The figure shows three views and two pictorial views of one solid part (mm, origin at its lowest corner). Answer the questions. A direction names the side the tool comes from. Give positions to 0.01 mm unless a question says otherwise; leave off trailing zeros. Write each loop counter-clockwise with the first axis right and the second up, starting at its lowest first coordinate (ties: lowest second). Pieces come first, ordered by that corner, then holes. Notation, with made-up numbers: (81.5, -9) - (139.5, -9) arc R23 ccw to (139.5, 15) - close; hole circle Ø2 at (85, 33). An arc over 180 degrees is marked (long way). Use CSV: the item, a comma, the result in double quotes. Start each with the question number.
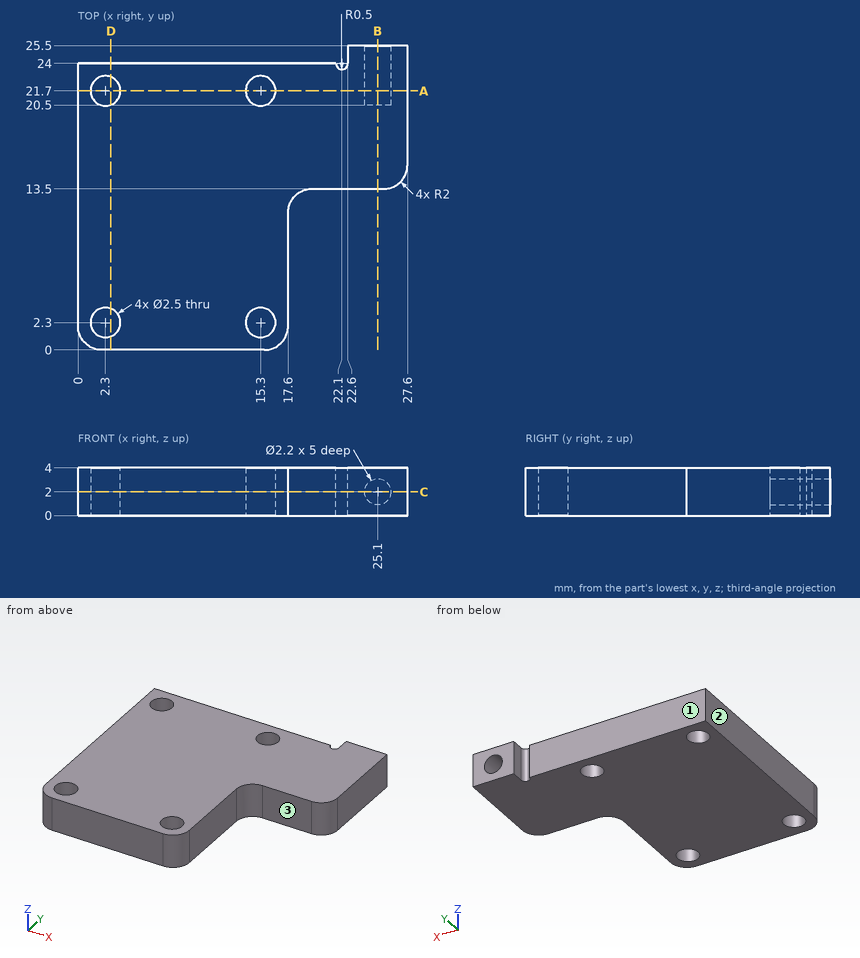
(1) The part is cut by section A-A on y = 21.7. Write down the section's boundary in (x, z), plus the area to 3 significant figures.
(2) The part is cut by section C-C on z = 2. Write down the section's boundary in (x, y), plus the area to 3 significant figures.
(3) The part is cut by section D-D on x = 2.75. Write down the section's boundary in (y, z), plus the area to 3 significant figures.
(4) The part is cut by section B-B on x = 25.1. Write down the section's boundary in (y, z), plus the area to 3 significant figures.
(5) Consider probe 1 along Y at (x, z) = (2.3, 2.7); probe 2 along X at (y, z) = (24.25, 2); probe 3 along X at (y, z) = (9.25, 0.65). Determine where each line is inside the solid, lowest interval first.
(6) Given P1, Ø1.5, axis at x = 19, z = 0.5, coming from the -Y side; P2, Ø2, axis at x = 15.3, y = 2.3, coming from the +Z side; P3, Ø1.8, axis at x = 25.1, z = 2, coming from the +Y side, each flat-ended and moving along its own axis, determine where each tip first touches the part or whether it passes through.
(7) Which of the six approach directions +Z, -Z, +X, -X, +Y, -Y give full straight-line access (tool end or side, diameter ignored) to the marked faces 1, 2 and 3?
Reported:
1,outline,"(0, 0) - (1.05, 0) - (1.05, 4) - (0, 4) - close; (3.55, 0) - (14.05, 0) - (14.05, 4) - (3.55, 4) - close; (16.55, 0) - (27.6, 0) - (27.6, 4) - (16.55, 4) - close; hole circle Ø2.2 at (25.1, 2)"
1,area,"86.6 mm²"
2,outline,"(0, 2) arc R2 ccw to (2, 0) - (15.6, 0) arc R2 ccw to (17.6, 2) - (17.6, 11.5) arc R2 cw to (19.6, 13.5) - (25.6, 13.5) arc R2 ccw to (27.6, 15.5) - (27.6, 25.5) - (26.2, 25.5) - (26.2, 20.5) - (24, 20.5) - (24, 25.5) - (22.6, 25.5) - (22.6, 24) arc R0.5 cw to (21.6, 24) - (0, 24) - close; hole circle Ø2.5 at (2.3, 2.3); hole circle Ø2.5 at (2.3, 21.7); hole circle Ø2.5 at (15.3, 2.3); hole circle Ø2.5 at (15.3, 21.7)"
2,area,"502 mm²"
3,outline,"(0, 0) - (1.13, 0) - (1.13, 4) - (0, 4) - close; (3.47, 0) - (20.53, 0) - (20.53, 4) - (3.47, 4) - close; (22.87, 0) - (24, 0) - (24, 4) - (22.87, 4) - close"
3,area,"77.3 mm²"
4,outline,"(13.5, 0) - (25.5, 0) - (25.5, 0.9) - (20.5, 0.9) - (20.5, 3.1) - (25.5, 3.1) - (25.5, 4) - (13.5, 4) - close"
4,area,"37.0 mm²"
5,probe 1,"0 to 1.05, 3.55 to 20.45, 22.95 to 24"
5,probe 2,"22.6 to 24, 26.2 to 27.6"
5,probe 3,"0 to 17.6"
6,P1,"y = 12.98"
6,P2,"through"
6,P3,"y = 20.5"
7,face 1,"+Z, -Z, -X, +Y"
7,face 2,"+Z, -Z, -X, +Y, -Y"
7,face 3,"+Z, -Z, +X, -Y"
